```python
from build123d import *

# Parameters (mm, degrees)
BOSS_EXTRUDE1_DEPTH     = 10
SKETCH2_W               = 17.2
SKETCH2_H               = 43
CUT_EXTRUDE1_DEPTH      = 72.414284285
SKETCH3_W               = 90
SKETCH3_H               = 34
SKETCH3_W_2             = 80
SKETCH3_H_2             = 24
BOSS_EXTRUDE3_DEPTH     = 15
SKETCH4_W               = 49.6
SKETCH4_H               = 5
BOSS_EXTRUDE4_DEPTH     = 10
SKETCH5_W               = 15
SKETCH5_H               = 22
BOSS_EXTRUDE5_DEPTH     = 5
SKETCH6_W               = 90
SKETCH6_H               = 77
BOSS_EXTRUDE6_DEPTH     = 15
BOSS_EXTRUDE8_DEPTH     = 39
CHAMFER1_SIZE           = 64
CHAMFER1_SIZE_2         = 3.354097874
CHAMFER2_SIZE           = 64
CHAMFER2_SIZE_2         = 11.405813635
CHAMFER3_SIZE           = 64
CHAMFER3_SIZE_2         = 13.775745352
CUT_EXTRUDE3_DEPTH      = 95.500525601
CUT_EXTRUDE3_DEPTH_BACK = 95.500525601
SKETCH10_W              = 50
SKETCH10_H              = 27
SKETCH15_R              = 8
CUT_EXTRUDE5_DEPTH      = 122.227059686
CUT_EXTRUDE6_DEPTH      = 2.5
SKETCH18_W              = 29.6
SKETCH18_H              = 43
CUT_EXTRUDE7_DEPTH      = 10
CUT_EXTRUDE8_DEPTH      = 15
SKETCH21_W              = 29.6
SKETCH21_H              = 33
BOSS_EXTRUDE10_DEPTH    = 4.5
SKETCH23_W              = 2.05
SKETCH23_H              = 13
BOSS_EXTRUDE11_DEPTH    = 15


with BuildPart() as part:
    # Sketch1 → Boss-Extrude1 (new body)
    with BuildSketch(Plane(origin=(0, 0, 0), x_dir=(1, 0, 0), z_dir=(0, 1, 0))):
        with BuildLine():
            Line((-35, 50), (35, 50))
            ThreePointArc((35, 50), (45.606601718, 45.606601718), (50, 35))
            Line((50, 35), (50, -35))
            ThreePointArc((50, -35), (45.606601718, -45.606601718), (35, -50))
            Line((35, -50), (-35, -50))
            ThreePointArc((-35, -50), (-45.606601718, -45.606601718), (-50, -35))
            Line((-50, -35), (-50, 35))
            ThreePointArc((-50, 35), (-45.606601718, 45.606601718), (-35, 50))
        make_face()
    extrude(amount=BOSS_EXTRUDE1_DEPTH)

    # Sketch2 → Cut-Extrude1 (cut, through all)
    with BuildSketch(Plane(origin=(0, 10, 0), x_dir=(1, 0, 0), z_dir=(0, 1, 0))):
        with Locations((-33.4, 18.5)):
            Rectangle(SKETCH2_W, SKETCH2_H)
        with Locations((33.4, 18.5)):
            Rectangle(SKETCH2_W, SKETCH2_H)
    extrude(amount=-CUT_EXTRUDE1_DEPTH, mode=Mode.SUBTRACT)

    # Sketch3 → Boss-Extrude3 (add)
    with BuildSketch(Plane(origin=(0, 10, 0), x_dir=(1, 0, 0), z_dir=(0, 1, 0))):
        with Locations((0, -20)):
            Rectangle(SKETCH3_W, SKETCH3_H)
        with Locations((0, -20)):
            Rectangle(SKETCH3_W_2, SKETCH3_H_2, mode=Mode.SUBTRACT)
    extrude(amount=BOSS_EXTRUDE3_DEPTH)

    # Sketch4 → Boss-Extrude4 (add)
    with BuildSketch(Plane(origin=(0, 10, 0), x_dir=(1, 0, 0), z_dir=(0, 1, 0))):
        with Locations((0, 10)):
            Rectangle(SKETCH4_W, SKETCH4_H)
        with Locations((0, 27)):
            Rectangle(SKETCH4_W, SKETCH4_H)
    extrude(amount=BOSS_EXTRUDE4_DEPTH)

    # Sketch5 → Boss-Extrude5 (add)
    with BuildSketch(Plane(origin=(0, 20, 0), x_dir=(1, 0, 0), z_dir=(0, 1, 0))):
        with Locations((-17.3, 18.5)):
            Rectangle(SKETCH5_W, SKETCH5_H)
        with Locations((17.3, 18.5)):
            Rectangle(SKETCH5_W, SKETCH5_H)
    extrude(amount=BOSS_EXTRUDE5_DEPTH)

    # Sketch6 → Boss-Extrude6 (add)
    with BuildSketch(Plane(origin=(0, 10, 0), x_dir=(1, 0, 0), z_dir=(0, 1, 0))):
        with BuildLine():
            Line((-50, 35), (-50, -35))
            ThreePointArc((-50, -35), (-45.606601718, -45.606601718), (-35, -50))
            Line((-35, -50), (35, -50))
            ThreePointArc((35, -50), (45.606601718, -45.606601718), (50, -35))
            Line((50, -35), (50, 35))
            ThreePointArc((50, 35), (45.606601718, 45.606601718), (35, 50))
            Line((35, 50), (-35, 50))
            ThreePointArc((-35, 50), (-45.606601718, 45.606601718), (-50, 35))
        make_face()
        with Locations((0, 1.5)):
            Rectangle(SKETCH6_W, SKETCH6_H, mode=Mode.SUBTRACT)
    extrude(amount=BOSS_EXTRUDE6_DEPTH)

    # Sketch9 → Boss-Extrude8 (add)
    with BuildSketch(Plane(origin=(0, 25, 0), x_dir=(1, 0, 0), z_dir=(0, 1, 0))):
        with BuildLine():
            Line((-50, 35), (-50, -35))
            ThreePointArc((-50, -35), (-45.606601718, -45.606601718), (-35, -50))
            Line((-35, -50), (35, -50))
            ThreePointArc((35, -50), (45.606601718, -45.606601718), (50, -35))
            Line((50, -35), (50, 35))
            ThreePointArc((50, 35), (45.606601718, 45.606601718), (35, 50))
            Line((35, 50), (-35, 50))
            ThreePointArc((-35, 50), (-45.606601718, 45.606601718), (-50, 35))
        make_face()
        with BuildLine():
            Line((-45, 35), (-45, -32))
            Line((-45, -32), (45, -32))
            Line((45, -32), (45, 35))
            ThreePointArc((45, 35), (44.659258263, 37.588190451), (43.660254038, 40))
            Line((43.660254038, 40), (-43.660254038, 40))
            ThreePointArc((-43.660254038, 40), (-44.659258263, 37.588190451), (-45, 35))
        make_face(mode=Mode.SUBTRACT)
    extrude(amount=BOSS_EXTRUDE8_DEPTH)

    # Chamfer1
    # the kernel refuses this chamfer: 64, 3.354097874 mm, written as the material it takes off along each edge
    with BuildSketch(Plane(origin=(-35, 64, 50), x_dir=(0, -0.9999979738662979, 0.002013023422382214), z_dir=(1, 0, 0)), Plane(origin=(50, 64, 35), x_dir=(0.002013023422382214, -0.9999979738662979, 0), z_dir=(0, 0, -1)), Plane(origin=(-50, 64, -35), x_dir=(-0.002013023422382214, -0.9999979738662979, 0), z_dir=(0, 0, 1)), Plane(origin=(35, 64, -50), x_dir=(0, -0.9999979738662979, -0.002013023422382214), z_dir=(-1, 0, 0))) as chamfer1_piece_1:
        Polygon((CHAMFER1_SIZE * 0.999997973866, CHAMFER1_SIZE * 0.00201302342238), (-CHAMFER1_SIZE_2 * 0.00201302342245, CHAMFER1_SIZE_2 * 0.9999979739), (0, 0), align=None)
    extrude(amount=70, mode=Mode.SUBTRACT)
    with BuildSketch(Plane(origin=(35, 64, 35), x_dir=(0, 0, 1), z_dir=(-1, 0, 0))) as chamfer1_piece_2:
        Polygon((15, -CHAMFER1_SIZE), (15 - CHAMFER1_SIZE_2, 0), (15, 0), align=None)
    revolve(axis=Axis((35, 64, 35), (0, 1, 0)), revolution_arc=90, mode=Mode.SUBTRACT)
    with BuildSketch(Plane(origin=(-35, 64, 35), x_dir=(-1, 0, 0), z_dir=(0, 0, -1))) as chamfer1_piece_3:
        Polygon((15, -CHAMFER1_SIZE), (15 - CHAMFER1_SIZE_2, 0), (15, 0), align=None)
    revolve(axis=Axis((-35, 64, 35), (0, 1, 0)), revolution_arc=90, mode=Mode.SUBTRACT)
    with BuildSketch(Plane(origin=(35, 64, -35), x_dir=(1, 0, 0), z_dir=(0, 0, 1))) as chamfer1_piece_4:
        Polygon((15, -CHAMFER1_SIZE), (15 - CHAMFER1_SIZE_2, 0), (15, 0), align=None)
    revolve(axis=Axis((35, 64, -35), (0, 1, 0)), revolution_arc=90, mode=Mode.SUBTRACT)
    with BuildSketch(Plane(origin=(-35, 64, -35), x_dir=(0, 0, -1), z_dir=(1, 0, 0))) as chamfer1_piece_5:
        Polygon((15 - CHAMFER1_SIZE_2, 0), (15, -CHAMFER1_SIZE), (15, 0), align=None)
    revolve(axis=Axis((-35, 64, -35), (0, 1, 0)), revolution_arc=90, mode=Mode.SUBTRACT)

    # Chamfer2
    # the kernel refuses this chamfer: 64, 11.405813635 mm, written as the material it takes off along each edge
    with BuildSketch(Plane(origin=(201.306482971, 64, -46.645902126), x_dir=(0, -0.9982575003065525, -0.05900816114499234), z_dir=(-1, 0, 0))) as chamfer2_piece_1:
        Polygon((CHAMFER2_SIZE * 0.999977671636, CHAMFER2_SIZE * 0.0066825316561), (-CHAMFER2_SIZE_2 * 0.0590081611462, CHAMFER2_SIZE_2 * 0.998257500326), (0, 0), align=None)
    extrude(amount=402.612965942, mode=Mode.SUBTRACT)

    # Chamfer3
    # the kernel refuses this chamfer: 64, 13.775745352 mm, written as the material it takes off along each edge
    with BuildSketch(Plane(origin=(-201.265469314, 64, 46.645902126), x_dir=(0, -0.9981787050157903, 0.06032638604292662), z_dir=(1, 0, 0))) as chamfer3_piece_1:
        Polygon((CHAMFER3_SIZE * 0.999967974892, CHAMFER3_SIZE * 0.00800307379952), (-CHAMFER3_SIZE_2 * 0.060326386045, CHAMFER3_SIZE_2 * 0.99817870505), (0, 0), align=None)
    extrude(amount=402.530938629, mode=Mode.SUBTRACT)

    # Sketch10 → Cut-Extrude3 (cut, two sides: drawn at the far end of the back side and taken through both)
    with BuildSketch(Plane(origin=(0, 1.307501734, 0), x_dir=(0, 0, 1), z_dir=(-1, 0, 0)).offset(-CUT_EXTRUDE3_DEPTH_BACK)):
        with Locations((-22.129843227, 49.192498266)):
            Rectangle(SKETCH10_W, SKETCH10_H)
    extrude(amount=CUT_EXTRUDE3_DEPTH + CUT_EXTRUDE3_DEPTH_BACK, mode=Mode.SUBTRACT)

    # Sketch15 → Cut-Extrude5 (cut, through all)
    with BuildSketch(Plane.XY.offset(-40)):
        with Locations((-12.75, 20.25)):
            Circle(SKETCH15_R)
        with Locations((12.75, 20.25)):
            Circle(SKETCH15_R)
    extrude(amount=-CUT_EXTRUDE5_DEPTH, mode=Mode.SUBTRACT)

    # Sketch17 → Cut-Extrude6 (cut)
    with BuildSketch(Plane(origin=(0, 0, -29.5), x_dir=(-1, 0, 0), z_dir=(0, 0, -1))):
        Polygon((-24.8, 10), (24.8, 10), (24.8, 25), (9.8, 25), (9.8, 20), (-9.8, 20), (-9.8, 25), (-24.8, 25), align=None)
    extrude(amount=-CUT_EXTRUDE6_DEPTH, mode=Mode.SUBTRACT)

    # Sketch18 → Cut-Extrude7 (cut)
    with BuildSketch(Plane.XZ):
        with Locations((0, -18.5)):
            Rectangle(SKETCH18_W, SKETCH18_H)
    extrude(amount=-CUT_EXTRUDE7_DEPTH, mode=Mode.SUBTRACT)

    # Sketch20 → Cut-Extrude8 (cut)
    with BuildSketch(Plane.XZ.offset(-25)):
        with BuildLine():
            Line((-45, -35), (-45, -40))
            Line((-45, -40), (-43.660254038, -40))
            ThreePointArc((-43.660254038, -40), (-44.659258263, -37.588190451), (-45, -35))
        make_face()
        with BuildLine():
            Line((45, -40), (45, -35))
            ThreePointArc((45, -35), (44.659258263, -37.588190451), (43.660254038, -40))
            Line((43.660254038, -40), (45, -40))
        make_face()
    extrude(amount=-CUT_EXTRUDE8_DEPTH, mode=Mode.SUBTRACT)

    # Sketch21 → Boss-Extrude10 (add)
    with BuildSketch(Plane.XZ):
        with Locations((0, -13.5)):
            Rectangle(SKETCH21_W, SKETCH21_H)
    extrude(amount=-BOSS_EXTRUDE10_DEPTH)

    # Sketch23 → Boss-Extrude11 (add)
    with BuildSketch(Plane(origin=(0, 10, 0), x_dir=(1, 0, 0), z_dir=(0, 1, 0))):
        with Locations((-23.775, 33.5)):
            Rectangle(SKETCH23_W, SKETCH23_H)
        with Locations((23.775, 33.5)):
            Rectangle(SKETCH23_W, SKETCH23_H)
    extrude(amount=BOSS_EXTRUDE11_DEPTH)


solid = part.part
```
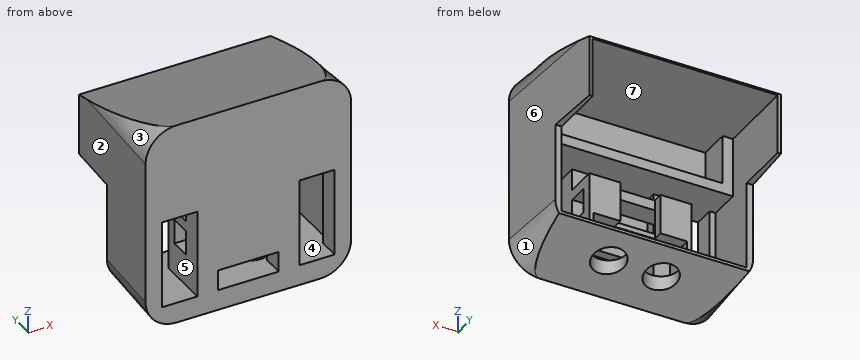
Check sheet for the modelled part. Datum: model origin and axes. Units: mm. Face numbers are marked on the shaded views. A direction names the side the tool comes from. Coordinates: 2 decimals unless noted, no trailing zeros. Loops run counter-clockwise (first coordinate to the right, second up) from the corner with the lowest first, then second, coordinate; pieces in that order, holes last. Notation, with made-up numbers: M 75,70 L 96,70 A32 ccw 96,106 Z; hole C 32.5,-29.75 d9. An arc over 180 degrees is marked long. Answer as a JSON object with one key per item and string values.
1. Scan lines: L1, parallel to X at y = 20.25, z = -45; L2, parallel to X at y = 20, z = -42; L3, parallel to Y at x = 17, z = -14. Record each from-to range of solid material in increasing order. Write a range as from..to.
Outcome:
{"L1": "-44.71..-20.75, -4.75..4.75, 20.75..44.71", "L2": "-47.07..-20.75, -4.75..4.75, 20.75..47.07", "L3": "0..10, 20..25"}
2. Release check for a two-part mould opening along Z. For the marked faces 1, 2, 3 and 4 record: pulls with the +Z half, pulls with the -Z half, needs draft (parallel to the pull), parting line crosses it, or undercut.
Outcome:
{"face 1": "pulls with the -Z half", "face 2": "needs draft", "face 3": "pulls with the +Z half", "face 4": "undercut"}
3. Sectioned sample at C-C on x = 12.75. Record the cut outline in (y, z), and give its area (3 significant figures).
Outcome:
{"outline": "M 0,-50 L 0.09,-50 L 12.25,-47.19 L 12.25,-40 L 0,-40 Z; M 0,-30 L 4.5,-30 L 4.5,3 L 25,3 L 25,8 L 10,8 L 10,32 L 64,32 L 64,32.87 L 0.09,50 L 0,50 Z; M 10,-27 L 25,-27 L 25,-7.5 L 10,-7.5 L 10,-12.5 L 20,-12.5 L 20,-24.5 L 10,-24.5 Z; M 28.25,-43.49 L 37,-41.47 L 37,-40 L 28.25,-40 Z", "area": "1,420 mm²"}
4. Sectioned sample at A-A on z = -22.5. Record the cut outline in (x, y), and give its area (3 significant figures).
Outcome:
{"outline": "M -50,0 L -42,0 L -42,10 L -45,10 L -45,37 L -48.06,37 Z; M -24.8,0 L 24.8,0 L 24.8,10 L 14.8,10 L 14.8,4.5 L -14.8,4.5 L -14.8,10 L -24.8,10 Z; M -24.8,20 L -9.8,20 L -9.8,25 L -24.8,25 Z; M 9.8,20 L 24.8,20 L 24.8,25 L 9.8,25 Z; M 42,0 L 50,0 L 48.06,37 L 45,37 L 45,10 L 42,10 Z", "area": "841 mm²"}
5. Depth check by flat-ended pin: P1, Ø19, axis at x = 14, z = 21.5, coming from the +Y side; P2, Ø3, axis at y = 37, z = -10, coming from the +X side; P3, Ø5, axis at y = 45, z = 18.5, coming from the -X side; P4, Ø3.5, axis at x = -17, z = -21.5, coming from the -Y side. Enter the tip coordinate at first touch or a pass-through.
Outcome:
{"P1": "y = 10", "P2": "x = 48.14", "P3": "x = -47.77", "P4": "y = 0"}
6. Access from +Z, -Z, +X, -X, +Y, -Y to the whole of each face (thin tool, end or side, straight path). Record for the marked faces 5, 6 and 7.
Outcome:
{"face 5": "+Y, -Y", "face 6": "+Z, -Z, +X, +Y", "face 7": "+Y"}
7. Sectioned sample at B-B on z = 22. Record the cut outline in (x, y), and give its area (3 significant figures).
Outcome:
{"outline": "M -50,0 L 50,0 L 46.65,64 L 45,64 L 45,25 L 40,25 L 40,10 L -40,10 L -40,25 L -45,25 L -45,64 L -46.65,64 Z", "area": "1,480 mm²"}
8. Sectioned sample at D-D on y = 31. Record the cut outline in (x, z).
Outcome:
{"outline": "M -48.38,-35 A13.38 ccw -45.82,-42.86 L 45.82,-42.86 A13.38 ccw 48.38,-35 L 48.38,35 A13.38 ccw 46.57,41.71 L -46.57,41.71 A13.38 ccw -48.38,35 Z; hole M -45,-40 L 45,-40 L 45,32 L -45,32 Z"}
